Read the model definition and answer for the solid it produces. Units are mm, in the model's axes. A direction names the side the tool comes from. Round coordinates to 2 decimals unless told otherwise and drop trailing zeros. Loops run counter-clockwise (first coordinate to the right, second up) from the corner with the lowest first, then second, coordinate; pieces in that order, holes last. Notation, with made-up numbers: M -6,-32 L 49,-32 A27 ccw 49,-10 Z; hole C 77,-37.75 d2. An arc over 180 degrees is marked long. Write each question's results on one line, items separated by ' | '.
Autodesk Fusion 360 part; units mm, degrees
sketch "Sketch1" plane through (0, 0, 0) normal (0, 1, 0) x (1, 0, 0)
  line L0 (-31.75, 12.7) -> (31.75, 12.7)
  line L1 (38.1, 6.35) -> (38.1, -6.35)
  line L2 (31.75, -12.7) -> (-31.75, -12.7)
  line L3 (-38.1, -6.35) -> (-38.1, 6.35)
  line L4 (38.1, -6.35) -> (38.1, -12.7)
  line L5 (38.1, -12.7) -> (31.75, -12.7)
  line L6 (38.1, 6.35) -> (38.1, 12.7)
  line L7 (38.1, 12.7) -> (31.75, 12.7)
  line L8 (-38.1, 6.35) -> (-38.1, 12.7)
  line L9 (-38.1, 12.7) -> (-31.75, 12.7)
  line L10 (-38.1, -6.35) -> (-38.1, -12.7)
  line L11 (-38.1, -12.7) -> (-31.75, -12.7)
  point P0 (-38.1, 12.7)
  point P1 (38.1, 12.7)
  point P2 (38.1, -12.7)
  point P3 (-38.1, -12.7)
extrude "Extrude1" add sketch "Sketch1" along normal blind 7.62
sketch "Sketch2" plane through (0, 7.62, 0) normal (0, 1, 0) x (-1, 0, 0)
  line L0 (38.1, -12.7) -> (38.1, 12.7)
  line L1 (38.1, 12.7) -> (-38.1, 12.7)
  line L2 (-38.1, 12.7) -> (-38.1, -12.7)
  line L3 (-38.1, -12.7) -> (38.1, -12.7)
  line L4 (-19.05, 12.7) -> (19.05, 12.7)
  line L5 (19.05, 12.7) -> (19.05, -12.7)
  line L6 (19.05, -12.7) -> (-19.05, -12.7)
  line L7 (-19.05, -12.7) -> (-19.05, 12.7)
  line L8 (-19.05, 12.7) -> (19.05, -12.7) construction
  line L9 (19.05, 12.7) -> (-19.05, -12.7) construction
  dimension "d12" = 38.1
extrude "Extrude2" add sketch "Sketch2" along normal blind 44.45 contours L1 L3 L4 L5 L6 L7
sketch "Sketch3" plane through (0, 0, 12.7) normal (0, 0, 1) x (1, 0, 0)
  line L0 (-38.1, 0) -> (38.1, 0)
  line L1 (38.1, 7.62) -> (19.05, 7.62)
  line L2 (19.05, 7.62) -> (19.05, 52.07)
  line L3 (19.05, 52.07) -> (-19.05, 52.07)
  line L4 (-19.05, 52.07) -> (-19.05, 7.62)
  circle A0 centre (0, 25.4) radius 10.8585
  line L5 (38.1, 0) -> (38.1, 7.62)
  line L6 (-19.05, 7.62) -> (-38.1, 7.62)
  line L7 (-38.1, 7.62) -> (-38.1, 0)
  dimension "d15" = 25.4
  dimension "d16" = 21.717
  dimension "d47" = 25.4
extrude "Extrude3" cut sketch "Sketch3" against normal blind 25.4 contours A0
sketch "Sketch4" plane through (0, 52.07, 0) normal (0, 1, 0) x (-1, 0, 0)
  line L0 (-19.05, -12.7) -> (19.05, -12.7)
  line L1 (19.05, -12.7) -> (19.05, 12.7)
  line L2 (19.05, 12.7) -> (-19.05, 12.7)
  line L3 (-19.05, 12.7) -> (-19.05, -12.7)
  line L4 (-1.905, -12.7) -> (1.905, -12.7)
  line L5 (1.905, -12.7) -> (1.905, 12.7)
  line L6 (1.905, 12.7) -> (-1.905, 12.7)
  line L7 (-1.905, 12.7) -> (-1.905, -12.7)
  line L8 (-1.905, -12.7) -> (1.905, 12.7) construction
  line L9 (1.905, -12.7) -> (-1.905, 12.7) construction
  dimension "d19" = 3.81
extrude "Extrude4" cut sketch "Sketch4" along normal up to surface contours L0 L2 L4 L5 L6 L7 end surface at (10.8045, 24.3188, -4.2333)
fillet "Fillet1" radius 1.524 1 edges at (19.05, 7.62, 0)
fillet "Fillet1" radius 1.524 1 edges at (-19.05, 7.62, 0)
chamfer "Chamfer1" distance 0.635 angle 45 34 edges at (-19.05, 30.607, -12.7) (-19.05, 30.607, 12.7) (-19.4964, 8.0664, 12.7) (-29.337, 7.62, 12.7) (-19.4964, 8.0664, -12.7) (-29.337, 7.62, -12.7) (19.4964, 8.0664, -12.7) (29.337, 7.62, -12.7) (19.05, 30.607, -12.7) (29.337, 7.62, 12.7) (19.4964, 8.0664, 12.7) (19.05, 30.607, 12.7) (0, 0, -12.7) (-38.1, 0, 0) (-38.1, 3.81, -12.7) (38.1, 3.81, -12.7) (38.1, 0, 0) (38.1, 7.62, 0) (-38.1, 7.62, 0) (38.1, 3.81, 12.7) (0, 0, 12.7) (-38.1, 3.81, 12.7) (1.905, 44.08, -12.7) (1.905, 44.08, 12.7) (-1.905, 52.07, 0) (-1.905, 44.08, 12.7) (-1.905, 44.08, -12.7) (-10.4775, 52.07, -12.7) (-19.05, 52.07, 0) (-10.4775, 52.07, 12.7) (10.4775, 52.07, -12.7) (1.905, 52.07, 0) (19.05, 52.07, 0) (10.4775, 52.07, 12.7)
chamfer "Chamfer3" distance 0.762 angle 45 2 edges at (0, 14.5415, -12.7) (0, 14.5415, 12.7)
ref_plane "WorkPlane1" through (0, 26.035, 0) normal (0, 0, -1) x (-1, 0, 0)
sketch "Sketch5" plane through (0, 7.62, 0) normal (0, 1, 0) x (-1, 0, 0)
  line L0 (37.465, 12.065) -> (20.574, 12.065)
  line L1 (20.574, 12.065) -> (20.574, -12.065)
  line L2 (20.574, -12.065) -> (37.465, -12.065)
  line L3 (37.465, -12.065) -> (37.465, 12.065)
  line L4 (38.1, -12.065) -> (38.1, 12.065)
  line L5 (-38.1, 12.065) -> (-38.1, -12.065)
  point P0 (28.575, 0)
  point P1 (-28.575, 0)
  dimension "d33" = 9.525
  dimension "d34" = 9.525
hole "Hole1" at (-28.575, 7.62, 0) at (28.575, 7.62, 0) direction (0, -1, 0) diameter 3.6576 end through all counterbore diameter 7.1374 counterbore depth 3.5052
hole "Hole2" at (19.05, 43.7629, 0) direction (-1, 0, 0) diameter 2.7686 depth 33.02 tip angle 118 counterbore diameter 7.1374 counterbore depth 3.5052
move_body "Move1" bodies 1 to x (1, 0, 0) y (0, 1, 0) z (0, 0, 1) at (-152.4, 0, 0)
move_body "Move2" bodies 1 to x (1, 0, 0) y (0, 1, 0) z (0, 0, 1) at (152.4, 0, 0)
Item 1: Flat-ended cylindrical pins translate along their axes: pin 1 (5.5 mm diameter, centred on y = 44.5, z = 0, fed in from +X); pin 2 (2 mm diameter, centred on x = -28.575, z = 0, fed in from -Y); pin 3 (12.5 mm diameter, centred on y = 45, z = 5.5, fed in from +X); pin 4 (13.5 mm diameter, centred on x = 30, z = -1.5, fed in from +Y). Find the tip coordinate at first contact, or state that the pin passes through.
Outcome:
pin 1: stops at x = 15.54 | pin 2: passes through | pin 3: stops at x = 19.05 | pin 4: stops at y = 7.62
Item 2: The mould has two halves that part along X. Classify faces 4 (the face through (19.33, 7.87, -12.32)), 5 (the face through (-9, 14, -12.7)), 6 (the face through (26.76, 2.03, -0.24)), 7 (the face through (-0.46, 14.42, 12.07)): pulls with the +X half, pulls with the -X half, needs draft (parallel to the pull), parting line crosses it, or undercut.
Outcome:
face 4: pulls with the +X half | face 5: needs draft | face 6: undercut | face 7: undercut
Item 3: For faces 1 (the face through (-1.905, 42, 0)), 2 (the face through (31, 7.62, -3)), 3 (the face through (25.037, 5.843, -0.465)), determine the directions among +Z, -Z, +X, -X, +Y, -Y from which every point of the face is accessible in a straight line to the end or side of a thin tool.
Outcome:
face 1: +Z, -Z, +Y | face 2: +Z, -Z, +X, +Y | face 3: +Y
Item 4: The part is cut by section C-C (y = 48.5). Determine the outline of the cut face in (x, z) (3 decimals).
Outcome:
outline: M -19.05,-12.065 L -18.415,-12.7 L -2.54,-12.7 L -1.905,-12.065 L -1.905,12.065 L -2.54,12.7 L -18.415,12.7 L -19.05,12.065 Z; M 1.905,-12.065 L 2.54,-12.7 L 18.415,-12.7 L 19.05,-12.065 L 19.05,12.065 L 18.415,12.7 L 2.54,12.7 L 1.905,12.065 Z
Item 5: The part is cut by section B-B (x = 0). Determine the outline of the cut face in (y, z) (1 decimal), plus the area to 3 significant figures.
Outcome:
outline: M 0,-12.1 L 0.6,-12.7 L 13.8,-12.7 L 14.5,-11.9 L 14.5,11.9 L 13.8,12.7 L 0.6,12.7 L 0,12.1 Z | area: 368 mm2
Item 6: Straight lines are drawn through the part: line 1 (X direction, y = 50, z = -0.75) (3 decimals); line 2 (Y direction, x = -5.75, z = 0); line 3 (Y direction, x = -23, z = 0.25). For each, find the intervals that lie inside material, in ascending order.
Outcome:
line 1: x = -19.05 to -1.905, 1.905 to 19.05 | line 2: y = 0 to 16.19, 34.61 to 42.38, 45.15 to 52.07 | line 3: y = 0 to 7.62
